Read the model definition and answer for the solid it produces. Units are mm, in the model's axes. Give positions to 0.01 mm unless a question says otherwise; leave off trailing zeros. Order: outer loops, then holes, each group sorted by start corner. A loop starts at its lowest first (then second) coordinate and runs counter-clockwise, first axis right, second up. Notation, with made-up numbers: (45.5, -13.75) - (74.5, -13.75) arc R23 ccw to (74.5, 15.25) - close; hole circle Ø7 at (-15, 34). An arc over 180 degrees is marked (long way). Write each question's results on one line, items separated by ' | '.
Autodesk Inventor part; units mm, degrees
ref_plane "YZ Plane" through (0, 0, 0) normal (1, 0, 0) x (0, 1, 0)
ref_plane "XZ Plane" through (0, 0, 0) normal (0, 1, 0) x (-1, 0, 0)
ref_plane "XY Plane" through (0, 0, 0) normal (0, 0, 1) x (1, 0, 0)
sketch "スケッチ1" plane through (0, 0, 0) normal (0, 0, 1) x (1, 0, 0)
  line L0 (14.5843, 13.35) -> (-14.5843, 13.35)
  line L1 (-14.5843, 13.35) -> (-16.35, 11.5843)
  line L2 (-16.35, 11.5843) -> (-16.35, -42.5843)
  line L3 (-16.35, -42.5843) -> (-14.5843, -44.35)
  line L4 (-14.5843, -44.35) -> (14.5843, -44.35)
  line L5 (14.5843, -44.35) -> (16.35, -42.5843)
  line L6 (16.35, -42.5843) -> (16.35, 11.5843)
  line L7 (16.35, 11.5843) -> (14.5843, 13.35)
  circle A0 centre (-13.5, 10.5) radius 2.4
  circle A1 centre (13.5, -41.5) radius 2.4
  circle A2 centre (-13.5, -41.5) radius 2.4
  circle A3 centre (13.5, -10.5) radius 1.35
  circle A4 centre (-13.5, -10.5) radius 1.35
  circle A5 centre (13.5, 10.5) radius 2.4
  circle A6 centre (0, 0) radius 13
  line L8 (18.75, 15.75) -> (18.75, -47.6913)
  line L9 (-83.25, 15.75) -> (16.75, 15.75)
  line L10 (-73.341, 13.75) -> (-73.341, 3.75)
  line L11 (18.75, 15.75) -> (-73.341, 15.75)
  line L12 (-73.341, 15.75) -> (-73.341, -47.6913)
  line L13 (-73.341, -47.6913) -> (18.75, -47.6913)
  line L14 (18.75, -47.6913) -> (18.75, 15.75)
  line L15 (-52.6233, -21.6557) -> (-51.2333, -20.6912)
  arc A7 (-51.2333, -20.6912) -> (-53.5136, -17.4049) centre (-48.341, -16.25) ccw
  line L16 (-53.5136, -17.4049) -> (-54.9036, -18.3694)
  arc A8 (-54.9036, -18.3694) -> (-54.9539, -18.6477) centre (-54.7896, -18.5337) ccw
  line L17 (-54.9539, -18.6477) -> (-52.9016, -21.6054)
  arc A9 (-52.9016, -21.6054) -> (-52.6233, -21.6557) centre (-52.7373, -21.4914) ccw
  circle A10 centre (-48.341, -16.25) radius 19.7
  circle A11 centre (0, 0) radius 14
  circle A12 centre (-48.341, -16.25) radius 21
  dimension "d0" = 28
  dimension "d1" = 42
extrude "押し出し1" add sketch "スケッチ1" along normal blind 1 contours L7 L6 L5 L4 L3 L2 L1 L0 A11 | L8 L13 L12 L10 L9 L11
(1) Consider probe 1 along X at (y, z) = (-5, 0.9); probe 2 along X at (y, z) = (0, 0.25); probe 3 along X at (y, z) = (-9.5, 0.5). Determine where each line is inside the solid, lowest interval first. Write a range as [from, to].
Conclusion:
probe 1: [-73.34, -66.07], [-30.61, -13.08], [13.08, 18.75] | probe 2: [-73.34, -61.64], [-35.04, -14], [14, 18.75] | probe 3: [-73.34, -68.23], [-28.46, -14.41], [-12.59, -10.28], [10.28, 12.59], [14.41, 18.75]
(2) Section D-D (y = -41.5) is taken. Give the vertices of the cut face in (x, z).
Conclusion:
outline: (-73.34, 0) - (-15.9, 0) - (-15.9, 1) - (-73.34, 1) - close; (-11.1, 0) - (11.1, 0) - (11.1, 1) - (-11.1, 1) - close; (15.9, 0) - (18.75, 0) - (18.75, 1) - (15.9, 1) - close
(3) Section C-C (y = -16.25) is taken. Give the vertices of the cut face in (x, z), plus the area to 3 significant figures.
Conclusion:
outline: (-73.34, 0) - (-69.34, 0) - (-69.34, 1) - (-73.34, 1) - close; (-27.34, 0) - (18.75, 0) - (18.75, 1) - (-27.34, 1) - close | area: 50.1 mm^2
(4) Section B-B (z = 0.4) is taken. State how many separate pieces and enclosed holes the cut face has, plus the area to 3 significant figures.
Conclusion:
separate pieces: 1 | enclosed holes: 8 | area: 3,760 mm^2
(5) Section A-A (x = 0) is taken. Give the vertices of the cut face in (y, z).
Conclusion:
outline: (-47.69, 0) - (-14, 0) - (-14, 1) - (-47.69, 1) - close; (14, 0) - (15.75, 0) - (15.75, 1) - (14, 1) - close
(6) The mould has two halves that part along X. Classify faces 1 (the face through (-14.02, -39.157, 0.493)), 2 (the face through (-28, -23, 0)): pulls with the +X half, pulls with the -X half, needs draft (parallel to the pull), parting line crosses it, or undercut.
Conclusion:
face 1: undercut | face 2: needs draft
